Check sheet for the modelled part. Datum: model origin and axes. Units: mm. Give positions to 0.01 mm unless a question says otherwise; leave off trailing zeros. Write each loop counter-clockwise with the first axis right and the second up, starting at its lowest first coordinate (ties: lowest second). Pieces come first, ordered by that corner, then holes. Notation, with made-up numbers: M 38.25,50.5 L 65.25,50.5 A15 cw 65.25,68.5 Z; hole C -37.5,23 d6. An arc over 180 degrees is marked long. Write item = value, one per line. Start each with the question number.
1) Scan lines: line 1 along X through (y, z) = (0.7, 352.5); line 2 along Z through (x, y) = (35, 0.25); line 3 along Z through (x, y) = (-188.5, 0.8). Record each from-to range of solid material in increasing order. Write a range as [from, to].
2) Cross-section at A-A, the plane x = -4. Record the cut outline in (y, z), plus the area to 3 significant figures.
3) Cross-section at B-B, the plane y = 1.5. Record the cut outline in (x, z), plus the area to 3 significant figures.
4) Go/stop test with flat-tipped pins: pin 1 (4.5 mm diameter, centred on x = -187.01, z = 352.5, fed in from +Y); pin 2 (0.6 mm diameter, centred on y = 1, z = 136.5, fed in from +X). Record where each tip stops, or that it passes through.
Autodesk Inventor part; units mm, degrees
ref_plane "YZ Plane" through (0, 0, 0) normal (1, 0, 0) x (0, 1, 0)
ref_plane "XZ Plane" through (0, 0, 0) normal (0, 1, 0) x (-1, 0, 0)
ref_plane "XY Plane" through (0, 0, 0) normal (0, 0, 1) x (1, 0, 0)
sketch "Esquisse1" plane through (0, 0, 0) normal (0, 1, 0) x (-1, 0, 0)
  line L0 (235, 367.5) -> (-235, 367.5)
  line L1 (-235, 367.5) -> (-235, -367.5)
  line L2 (-235, -367.5) -> (235, -367.5)
  line L3 (235, -367.5) -> (235, 367.5)
  line L4 (235, 367.5) -> (-235, -367.5) construction
  line L5 (-235, 367.5) -> (235, -367.5) construction
  line L6 (227.0068, 355) -> (-227.0068, 355)
  line L7 (-227.0068, -355) -> (227.0068, -355)
  line L8 (227.0068, -355) -> (227.0068, 355)
  line L9 (227.0068, 355) -> (-227.0068, -355) construction
  line L10 (-227.0068, 355) -> (227.0068, -355) construction
  line L11 (122.9932, 195) -> (-227.0068, 195)
  line L12 (-227.0068, 195) -> (-227.0068, 45)
  line L13 (-227.0068, 45) -> (122.9932, 45)
  line L14 (122.9932, 45) -> (122.9932, 195)
  line L15 (122.9932, 195) -> (-227.0068, 45) construction
  line L16 (-227.0068, 195) -> (122.9932, 45) construction
  circle A0 centre (-187.0068, -352.5) radius 2.5
  circle A1 centre (187.0068, -352.5) radius 2.5
  circle A2 centre (187.0068, 30) radius 2.5
  circle A3 centre (-187.0068, 30) radius 2.5
  circle A4 centre (-187.0068, 352.5) radius 2.5
  circle A5 centre (187.0068, 352.5) radius 2.5
  line L17 (-227.0068, -355) -> (-197.0068, -355)
  line L18 (-227.0068, -325) -> (-227.0068, -355)
  line L19 (-227.0068, 45) -> (-235, 45)
  line L20 (-227.0068, 195) -> (-235, 195)
  line L21 (-227.0068, 355) -> (-227.0068, 195)
  line L22 (-227.0068, 45) -> (-227.0068, -355)
  point P0 (0, 0)
  point P1 (-52.0068, 120)
  dimension "d0" = 735
  dimension "d1" = 470
  dimension "d2" = 12.5
  dimension "d3" = 160
  dimension "d4" = 150
  dimension "d5" = 350
  dimension "d6" = 5
  dimension "d7" = 5
  dimension "d8" = 5
  dimension "d9" = 5
  dimension "d10" = 5
  dimension "d11" = 5
  dimension "d16" = 40
  dimension "d17" = 40
  dimension "d21" = 40
  dimension "d22" = 397.5
  dimension "d23" = 397.5
extrude "Extrusion1" add sketch "Esquisse1" along normal blind 2 contours L3 L2 L1 L19 L22 L18 L7 L8 L6 L21 L20 L0 | L21 L6 L8 L7 L18 L22 L13 L14 L11
properties part number "PlaqueSupperieur"
Reply:
q1.line_1 = [-235, -189.51], [-184.51, 184.51], [189.51, 235]
q1.line_2 = [-367.5, 45], [195, 367.5]
q1.line_3 = [-367.5, -354.51], [-350.49, 27.99], [32.01, 350.49], [354.51, 367.5]
q2.outline = M 0,-367.5 L 2,-367.5 L 2,45 L 0,45 Z; M 0,195 L 2,195 L 2,367.5 L 0,367.5 Z
q2.area = 1,170 mm2
q3.outline = M -235,-367.5 L 235,-367.5 L 235,45 L -122.99,45 L -122.99,195 L 235,195 L 235,367.5 L -235,367.5 Z; hole C -187.01,-352.5 d5; hole C -187.01,30 d5; hole C -187.01,352.5 d5; hole C 187.01,-352.5 d5; hole C 187.01,30 d5; hole C 187.01,352.5 d5
q3.area = 292,000 mm2
q4.pin_1 = through
q4.pin_2 = -122.99
